Read the model definition and answer for the solid it produces. Units are mm, in the model's axes. Coordinates: 2 decimals unless noted, no trailing zeros. Loops run counter-clockwise (first coordinate to the right, second up) from the corner with the lowest first, then second, coordinate; pieces in that order, holes last. Notation, with made-up numbers: M -29,-28 L -17,-28 A37 ccw -17,8 Z; hole C -40,58 d10. An arc over 180 degrees is marked long. Use one line per item in the form item = value. Start each with the question number.
1. Find the intervals of material crossed by probe 1 along Z at (x, y) = (-13.5, 0.75); probe 2 along X at (y, z) = (2.3, 31); probe 3 along Z at (x, y) = (-12, 2.4), in increasing order. Write a range as [from, to].
2. The part is cut by section D-D (x = -12). Give the number of separate pieces and of enclosed holes in the cut face, plus the area to 3 significant figures.
3. Flat-ended cylindrical pins translate along their axes: pin 1 (1.5 mm diameter, centred on x = -6.5, z = -28, fed in from -Y); pin 2 (5 mm diameter, centred on x = 12, z = 49, fed in from -Y). Find the tip coordinate at first contact, or state that the pin passes through.
4. The part is cut by section C-C (x = -1). Give the vertices of the cut face in (y, z).
5. The part is cut by section A-A (z = -56.75). Give the vertices of the cut face in (x, y), plus the area to 3 significant figures.
6. The part is cut by section B-B (x = 10). Give the vertices of the cut face in (y, z).
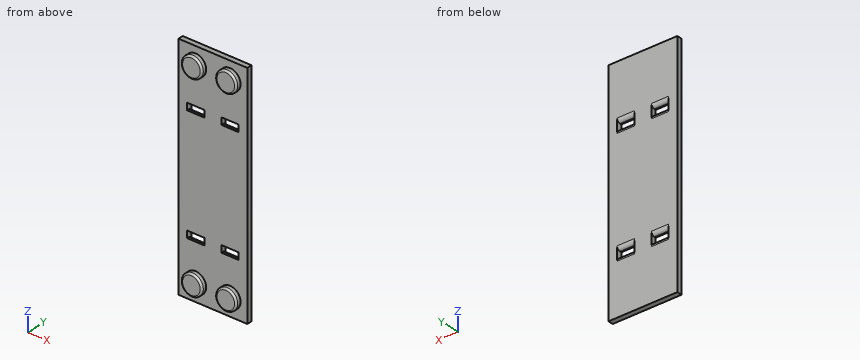
from build123d import *

# Parameters (mm, degrees)
SKETCH1_W           = 40
SKETCH1_H           = 133.5
BOSS_EXTRUDE1_DEPTH = 3
SKETCH2_R           = 6.11
BOSS_EXTRUDE2_DEPTH = 3
CUT_EXTRUDE1_REACH  = 71.94
SKETCH3_W           = 10
SKETCH3_H           = 4
FILLET3_R           = 1
FILLET4_R           = 2


with BuildPart() as part:
    # Sketch1 → Boss-Extrude1 (new body)
    with BuildSketch(Plane(origin=(0, 0, 0), x_dir=(1, 0, 0), z_dir=(0, 1, 0))):
        Rectangle(SKETCH1_W, SKETCH1_H)
    extrude(amount=BOSS_EXTRUDE1_DEPTH)

    # Sketch2 → Boss-Extrude2 (add)
    with BuildSketch(Plane.XZ):
        with Locations(Location((10, 56.75, 0), (0, 0, 90))):
            Circle(SKETCH2_R)
        with Locations(Location((-10, 56.75, 0), (0, 0, 90))):
            Circle(SKETCH2_R)
        with Locations(Location((-10, -56.75, 0), (0, 0, 90))):
            Circle(SKETCH2_R)
        with Locations(Location((10, -56.75, 0), (0, 0, 90))):
            Circle(SKETCH2_R)
    extrude(amount=BOSS_EXTRUDE2_DEPTH)

    # Sketch3 → Cut-Extrude1 (cut, up to next)
    with BuildSketch(Plane(origin=(0, 3, 0), x_dir=(1, 0, 0), z_dir=(0, 1, 0)), mode=Mode.PRIVATE) as cut_extrude1_sk1:
        with Locations((10, 33.3125)):
            Rectangle(SKETCH3_W, SKETCH3_H)
    cut_extrude1_tool1 = extrude(cut_extrude1_sk1.sketch, amount=-CUT_EXTRUDE1_REACH, mode=Mode.PRIVATE) & part.part
    # Sketch3 → Cut-Extrude1 (cut, up to next)
    with BuildSketch(Plane(origin=(0, 3, 0), x_dir=(1, 0, 0), z_dir=(0, 1, 0)), mode=Mode.PRIVATE) as cut_extrude1_sk2:
        with Locations((-10, 33.3125)):
            Rectangle(SKETCH3_W, SKETCH3_H)
    cut_extrude1_tool2 = extrude(cut_extrude1_sk2.sketch, amount=-CUT_EXTRUDE1_REACH, mode=Mode.PRIVATE) & part.part
    # Sketch3 → Cut-Extrude1 (cut, up to next)
    with BuildSketch(Plane(origin=(0, 3, 0), x_dir=(1, 0, 0), z_dir=(0, 1, 0)), mode=Mode.PRIVATE) as cut_extrude1_sk3:
        with Locations((-10, -33.3125)):
            Rectangle(SKETCH3_W, SKETCH3_H)
    cut_extrude1_tool3 = extrude(cut_extrude1_sk3.sketch, amount=-CUT_EXTRUDE1_REACH, mode=Mode.PRIVATE) & part.part
    # Sketch3 → Cut-Extrude1 (cut, up to next)
    with BuildSketch(Plane(origin=(0, 3, 0), x_dir=(1, 0, 0), z_dir=(0, 1, 0)), mode=Mode.PRIVATE) as cut_extrude1_sk4:
        with Locations((10, -33.3125)):
            Rectangle(SKETCH3_W, SKETCH3_H)
    cut_extrude1_tool4 = extrude(cut_extrude1_sk4.sketch, amount=-CUT_EXTRUDE1_REACH, mode=Mode.PRIVATE) & part.part
    add(cut_extrude1_tool1.solids().sort_by_distance((10, 3, -33.3125))[0], mode=Mode.SUBTRACT)
    add(cut_extrude1_tool2.solids().sort_by_distance((-10, 3, -33.3125))[0], mode=Mode.SUBTRACT)
    add(cut_extrude1_tool3.solids().sort_by_distance((-10, 3, 33.3125))[0], mode=Mode.SUBTRACT)
    add(cut_extrude1_tool4.solids().sort_by_distance((10, 3, 33.3125))[0], mode=Mode.SUBTRACT)

    # Fillet3
    fillet3_edges = [part.edges().sort_by_distance(p)[0] for p in [
        (10, -3, -62.86),
        (-10, -3, -62.86),
        (-10, -3, 50.64),
        (10, -3, 50.64),
    ]]
    fillet(fillet3_edges, radius=FILLET3_R)

    # Fillet4
    fillet4_edges = [part.edges().sort_by_distance(p)[0] for p in [
        (10, 3, 35.3125),
        (10, 3, 31.3125),
        (-10, 3, 35.3125),
        (-10, 3, 31.3125),
        (-10, 3, -35.3125),
        (-10, 3, -31.3125),
        (10, 3, -35.3125),
        (10, 3, -31.3125),
    ]]
    fillet(fillet4_edges, radius=FILLET4_R)


solid = part.part
Computed values:
q1.probe_1 = [-66.75, -35.31], [-31.31, 31.31], [35.31, 66.75]
q1.probe_2 = [-20, -15], [-5, 5], [15, 20]
q1.probe_3 = [-66.75, -35.88], [-30.74, 30.74], [35.88, 66.75]
q2.separate_pieces = 3
q2.enclosed_holes = 0
q2.area = 441 mm²
q3.pin_1 = 0
q3.pin_2 = -2.92
q4.outline = M 0,-66.75 L 3,-66.75 L 3,66.75 L 0,66.75 Z
q5.outline = M -20,0 L -16.11,0 L -16.11,-2 A1 ccw -15.11,-3 L -4.89,-3 A1 ccw -3.89,-2 L -3.89,0 L 3.89,0 L 3.89,-2 A1 ccw 4.89,-3 L 15.11,-3 A1 ccw 16.11,-2 L 16.11,0 L 20,0 L 20,3 L -20,3 Z
q5.area = 192 mm²
q6.outline = M -3,-61.86 A1 ccw -2,-62.86 L 0,-62.86 L 0,-66.75 L 3,-66.75 L 3,-37.31 A2 ccw 1,-35.31 L 0,-35.31 L 0,-50.64 L -2,-50.64 A1 ccw -3,-51.64 Z; M -3,51.64 A1 ccw -2,50.64 L 0,50.64 L 0,35.31 L 1,35.31 A2 ccw 3,37.31 L 3,66.75 L 0,66.75 L 0,62.86 L -2,62.86 A1 ccw -3,61.86 Z; M 0,-31.31 L 1,-31.31 A2 ccw 3,-29.31 L 3,29.31 A2 ccw 1,31.31 L 0,31.31 Z
